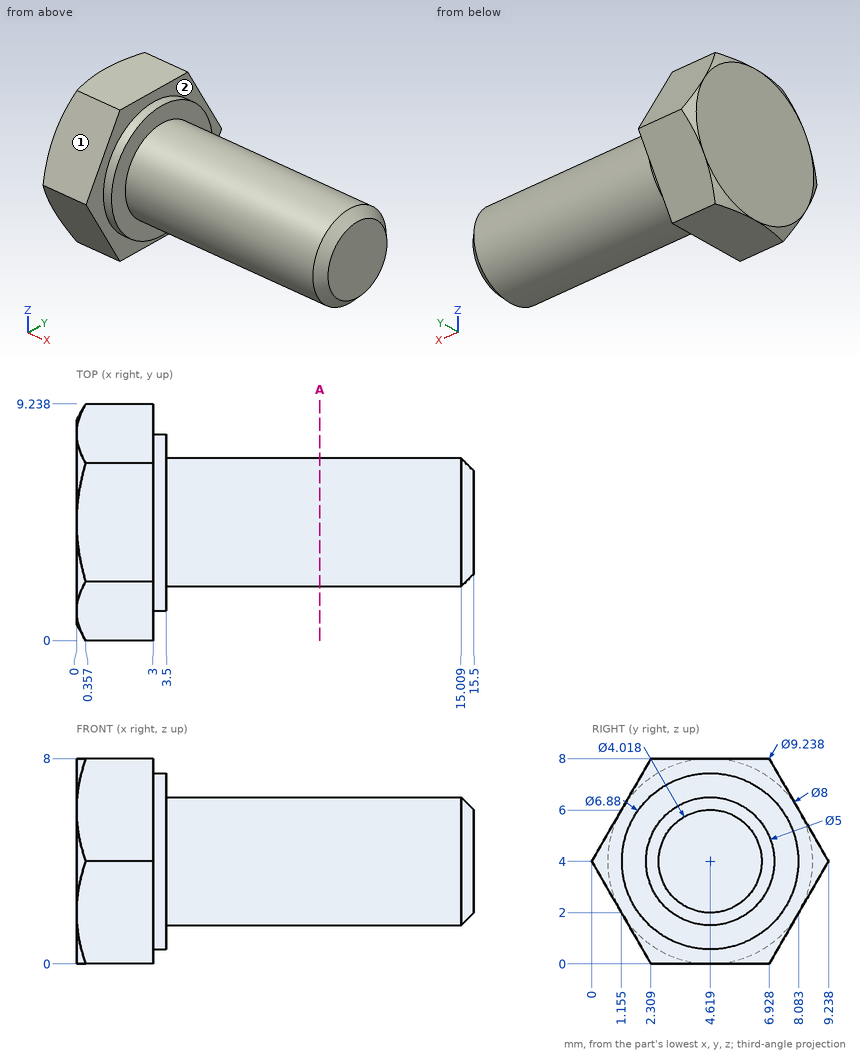
Geometry check sheet. Reference: drawing and pictorial views, mm from the part's lowest x, y, z. A direction names the side the tool comes from. Coordinates: 2 decimals unless noted, no trailing zeros. Order: outer loops, then holes, each group sorted by start corner. A loop starts at its lowest first (then second) coordinate and runs counter-clockwise, first axis right, second up. Notation, with made-up numbers: M 5.25,72 L 39.25,72 A22 ccw 39.25,104 Z; hole C 63.25,11 d1. An arc over 180 degrees is marked long. Return JSON: item names as keys, results as strings.
1) Thickness scan on L1, parallel to X at y = 6.75, z = 0.75; L2, parallel to X at y = 2, z = 5.75; L3, parallel to Z at x = 12.25, y = 4.75. Record the ranges inside material, lowest first. Write a range as [from, to].
Answer list:
{"L1": "[0, 3]", "L2": "[0, 3.5]", "L3": "[1.5, 6.5]"}
2) Gauge pin test, flat end, axial feed: pin 1 (1 mm diameter, centred on x = 11.5, y = 6, fed in from -Z). Record the tip position at first contact, or that the pin passes through.
Answer list:
{"pin 1": "z = 1.66"}
3) Cross-section at A-A, the plane x = 9.5. Record the boundary of the cut face in (y, z).
Answer list:
{"outline": "C 4.62,4 d5"}
4) Access from +Z, -Z, +X, -X, +Y, -Y to the whole of each face (thin tool, end or side, straight path). Record for the marked faces 1 and 2.
Answer list:
{"face 1": "+Z, +X, -X, -Y", "face 2": "+X"}
